Study the drawing (mm; zero at the part's minimum x, y, z) and answer. Coordinates: 2 decimals unless noted, no trailing zeros. Order: outer loops, then holes, each group sorted by start corner. A loop starts at its lowest first (then second) coordinate and runs counter-clockwise, first axis right, second up. Notation, with made-up numbers: (-30.75, 58) -> (9.25, 58) arc R36 ccw to (9.25, 94) -> close; hole circle Ø6 at (54.25, 63). An arc over 180 degrees is marked (long way). Write each question's results on one line, items separated by ' | '. Start each with the question number.
(1) Given pin 1 (0.6 mm diameter, centred on x = 73, z = 1, fed in from +Y); pin 2 (0.6 mm diameter, centred on x = 74, z = 1, fed in from -Y); pin 3 (0.6 mm diameter, centred on x = 58.5, z = 1.5, fed in from -Y), each flat-ended and moving along its own axis, determine where each tip first touches the part or whether it passes through.
(2) The part is cut by section D-D, the plane y = 68. Give the vertices of the cut face in (x, z).
(3) The part is cut by section B-B, the plane x = 67. Give the vertices of the cut face in (y, z), then the cut area to 3 significant figures.
(4) The part is cut by section A-A, the plane y = 23. Give the vertices of the cut face in (x, z), then the cut area to 3 significant figures.
(5) The part is cut by section C-C, the plane z = 1.4. Give the vertices of the cut face in (x, y), then the cut area to 3 significant figures.
(6) Straight lines are drawn through the part: L1, parallel to Y at x = 67, z = 0.85; L2, parallel to Y at x = 16.5, z = 0.7; L3, parallel to X at y = 68, z = 1.05. For each, find the intervals that lie inside material, in ascending order.
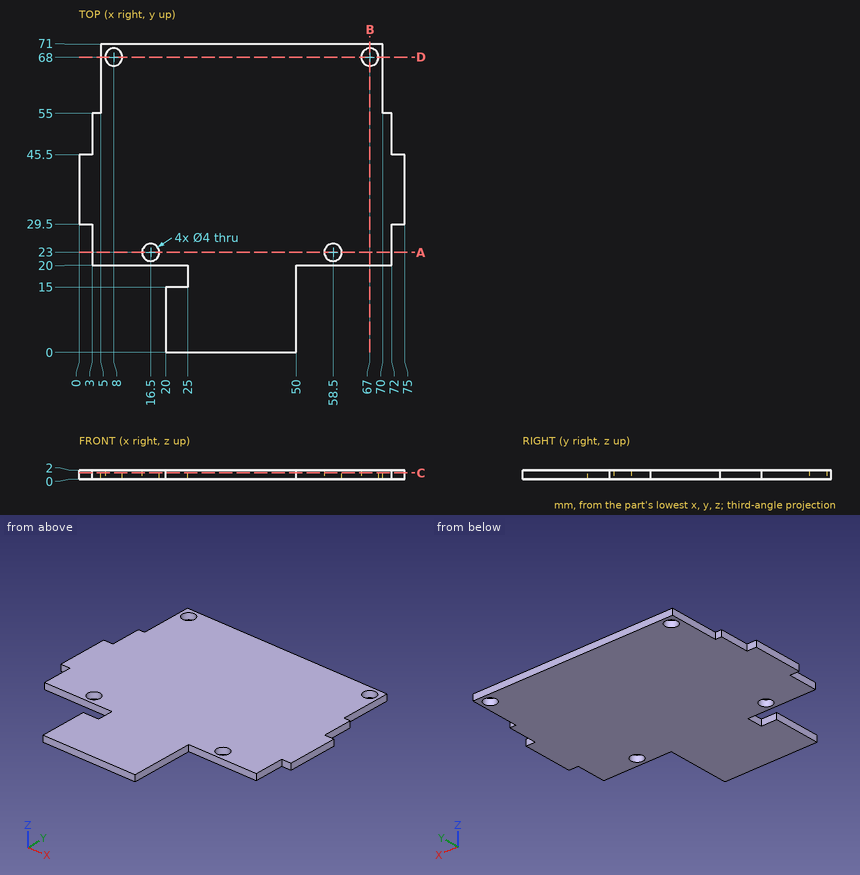
Established:
1) pin 1: stops at y = 45.5 | pin 2: stops at y = 29.5 | pin 3: stops at y = 20
2) outline: (5, 0) -> (6, 0) -> (6, 2) -> (5, 2) -> close; (10, 0) -> (65, 0) -> (65, 2) -> (10, 2) -> close; (69, 0) -> (70, 0) -> (70, 2) -> (69, 2) -> close
3) outline: (20, 0) -> (66, 0) -> (66, 2) -> (20, 2) -> close; (70, 0) -> (71, 0) -> (71, 2) -> (70, 2) -> close | area: 94.0 mm^2
4) outline: (3, 0) -> (14.5, 0) -> (14.5, 2) -> (3, 2) -> close; (18.5, 0) -> (56.5, 0) -> (56.5, 2) -> (18.5, 2) -> close; (60.5, 0) -> (72, 0) -> (72, 2) -> (60.5, 2) -> close | area: 122 mm^2
5) outline: (0, 29.5) -> (3, 29.5) -> (3, 20) -> (25, 20) -> (25, 15) -> (20, 15) -> (20, 0) -> (50, 0) -> (50, 20) -> (72, 20) -> (72, 29.5) -> (75, 29.5) -> (75, 45.5) -> (72, 45.5) -> (72, 55) -> (70, 55) -> (70, 71) -> (5, 71) -> (5, 55) -> (3, 55) -> (3, 45.5) -> (0, 45.5) -> close; hole circle Ø4 at (8, 68); hole circle Ø4 at (16.5, 23); hole circle Ø4 at (58.5, 23); hole circle Ø4 at (67, 68) | area: 4,080 mm^2
6) L1: y = 20 to 66, 70 to 71 | L2: y = 20 to 21, 25 to 71 | L3: x = 5 to 6, 10 to 65, 69 to 70
